Build history of the part. All positions in model axes, mm. A direction names the side the tool comes from. Coordinates: 2 decimals unless noted, no trailing zeros. Write each loop counter-clockwise with the first axis right and the second up, starting at its lowest first coordinate (ties: lowest second). Pieces come first, ordered by that corner, then holes.
```python
from build123d import *

# Parameters (mm, degrees)
PAD_DEPTH       = 20
SKETCH001_R     = 2.25
POCKET_DEPTH    = 2.5
SKETCH002_R     = 2.25
POCKET001_DEPTH = 2.5
FILLET_R        = 5
CHAMFER_SIZE    = 0.75


with BuildPart() as part:
    # Sketch → Pad (new body)
    with BuildSketch(Plane.XY):
        with BuildLine():
            Line((0, 0), (0, -50))
            Line((-27.500003, -50), (0, -50))
            ThreePointArc((-52.5, -25.000001), (-45.17767, -42.677669), (-27.500003, -50))
            Line((-52.5, -25.000001), (-52.5, 0))
            Line((-52.5, 2.5), (-52.5, 0))
            ThreePointArc((-2.5, 52.5), (-37.855339, 37.855339), (-52.5, 2.5))
            Line((0, 52.5), (-2.5, 52.5))
            Line((85.499965, 52.5), (0, 52.5))
            ThreePointArc((110.5, 27.499999), (103.177657, 45.177682), (85.499965, 52.5))
            Line((110.5, -25), (110.5, 27.499999))
            Line((108, -25), (110.5, -25))
            Line((108, 0), (108, -25))
            Line((0, 0), (108, 0))
        make_face()
        with BuildLine():
            Line((-2.5, 0), (-2.5, -47.5))
            Line((-27.5, -47.5), (-2.5, -47.5))
            ThreePointArc((-50, -25), (-43.409903, -40.909903), (-27.5, -47.5))
            Line((-50, 0), (-50, -25))
            Line((-2.5, 0), (-50, 0))
        make_face(mode=Mode.SUBTRACT)
        with BuildLine():
            Line((0, 2.5), (108, 2.5))
            Line((108, 2.5), (108, 27.5))
            ThreePointArc((108, 27.5), (101.409903, 43.409903), (85.5, 50))
            Line((85.5, 50), (0, 50))
            Line((0, 50), (0, 2.5))
        make_face(mode=Mode.SUBTRACT)
        with BuildLine():
            ThreePointArc((-2.5, 50), (-36.087572, 36.087572), (-50, 2.5))
            Line((-2.5, 2.5), (-50, 2.5))
            Line((-2.5, 50), (-2.5, 2.5))
        make_face(mode=Mode.SUBTRACT)
    extrude(amount=PAD_DEPTH)

    # Sketch001 (on Face7 of Pad) → Pocket (cut)
    with BuildSketch(Plane.YZ):
        with Locations((-37.5, 10)):
            Circle(SKETCH001_R)
        with Locations((-12.5, 10)):
            Circle(SKETCH001_R)
    extrude(amount=-POCKET_DEPTH, mode=Mode.SUBTRACT)

    # Sketch002 (on Face5 of Pad) → Pocket001 (cut)
    with BuildSketch(Plane(origin=(108, 0, 0), x_dir=(0, -1, 0), z_dir=(-1, 0, 0))):
        with Locations((12.5, 10)):
            Circle(SKETCH002_R)
    extrude(amount=-POCKET001_DEPTH, mode=Mode.SUBTRACT)

    # Fillet
    fillet_edges = [part.edges().sort_by_distance(p)[0] for p in [
        (109.25, -25, 0),
        (109.25, -25, 20),
    ]]
    fillet(fillet_edges, radius=FILLET_R)

    # Chamfer
    chamfer_edges = [part.edges().sort_by_distance(p)[0] for p in [
        (-37.855339, 37.855339, 20),
        (-37.855339, 37.855339, 0),
    ]]
    chamfer(chamfer_edges, length=CHAMFER_SIZE)


solid = part.part
```
1. Probe line 1 along X through (y, z) = (-15.5, 15.25); line 2 along Z through (x, y) = (-1.85, -37.5); line 3 along X through (y, z) = (43, 11.25). List the from-to ranges inside material, lowest first.
Computed values:
line 1: x = -52.5 to -50, -2.5 to 0, 108 to 110.5
line 2: z = 0 to 7.75, 12.25 to 20
line 3: x = -31.82 to -27.32, -2.5 to 0, 101.81 to 105.12
2. Mould opens along Z. For faces 1 (the face through (-1.232, -36.29, 11.897)), 2 (the face through (-37.024, 37.791, 19.88)), 3 (the face through (53, 2.5, 10)) say: +Z half, -Z half, draft (parallel to the pull), parting line (faces both ways), or undercut.
Computed values:
face 1: undercut
face 2: +Z half
face 3: draft
3. Saw through at C-C on z = 10. State how many separate pieces and enclosed holes the cut face has, plus the area to 3 significant figures.
Computed values:
separate pieces: 3
enclosed holes: 2
area: 1,470 mm2
4. Saw through at B-B on y = -12.5. List the corners of the cut face in (x, z), plus the area to 3 significant figures.
Computed values:
outline: (-52.5, 0.75) - (-51.75, 0) - (-50, 0) - (-50, 20) - (-51.75, 20) - (-52.5, 19.25) - close; (-2.5, 0) - (0, 0) - (0, 7.75) - (-2.5, 7.75) - close; (-2.5, 12.25) - (0, 12.25) - (0, 20) - (-2.5, 20) - close; (108, 0) - (109.75, 0) - (110.5, 0.75) - (110.5, 7.75) - (108, 7.75) - close; (108, 12.25) - (110.5, 12.25) - (110.5, 19.25) - (109.75, 20) - (108, 20) - close
area: 126 mm2
5. Flat gauge pins, fed straight in: pin 1 (2 mm diameter, centred on x = -32.5, z = 12.5, fed in from +Y); pin 2 (5 mm diameter, centred on y = -29.5, z = 5.5, fed in from +X); pin 3 (0.9 mm diameter, centred on x = 109, z = 8, fed in from -Y). Where does each tip first touch, or does it go through?
Computed values:
pin 1: stops at y = 43.23
pin 2: stops at x = 0
pin 3: stops at y = -25
6. 3-axis set-ups, long thin cutter, end or side, ignore diameter. For faces 4 (the face through (101.584, 43.234, 9.86)), 5 (the face through (109, -23, 19)), 6 (the face through (-14, -50, 10)), 7 (the face through (109, -23, 1)), 8 (the face through (53, 0, 10)): which of +Z, -Z, +X, -X, +Y, -Y reach the whole face in a straight line?
Computed values:
face 4: +Z, -Z
face 5: +Z, +X, -Y
face 6: +Z, -Z, +X, -X, -Y
face 7: -Z, +X, -Y
face 8: +Z, -Z, -Y
7. Saw through at A-A on x = 79. List the corners of the cut face in (y, z), plus the area to 3 significant figures.
Computed values:
outline: (0, 0) - (2.5, 0) - (2.5, 20) - (0, 20) - close; (50, 0) - (51.75, 0) - (52.5, 0.75) - (52.5, 19.25) - (51.75, 20) - (50, 20) - close
area: 99.4 mm2
